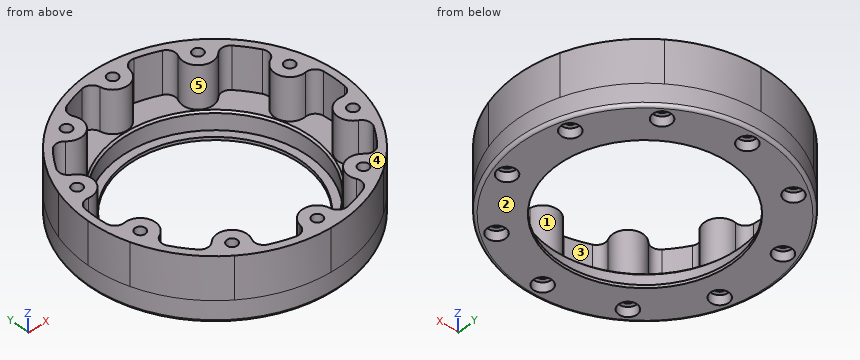
from build123d import *
from build123d.topology import SkipClean

# Parameters (mm, degrees)
ESQUISSE1_R             = 42
ESQUISSE1_R_2           = 31.2
BOSS_EXTRU_1_DEPTH      = 6
BOSS_EXTRU_2_START      = 1
ESQUISSE2_R             = 42
ESQUISSE2_R_2           = 28.6
BOSS_EXTRU_2_DEPTH      = 1
ESQUISSE3_R             = 5
BOSS_EXTRU_3_DEPTH      = 14
ESQUISSE4_R             = 42
ESQUISSE4_R_2           = 39.6
BOSS_EXTRU_4_DEPTH      = 14
CONG_1_R                = 3
ESQUISSE5_R             = 1.7
ENL_V_MAT_EXTRU_1_DEPTH = 64.000000167
ESQUISSE6_R             = 3
ENL_V_MAT_EXTRU_2_DEPTH = 3.2
CHANFREIN1_SIZE         = 0.6
CONG_2_R                = 1


with BuildPart() as part:
    # Esquisse1 → Boss.-Extru.1 (new body)
    with BuildSketch(Plane.XY):
        Circle(ESQUISSE1_R)
        Circle(ESQUISSE1_R_2, mode=Mode.SUBTRACT)
    extrude(amount=BOSS_EXTRU_1_DEPTH)

    # Esquisse2 → Boss.-Extru.2 (add)
    with BuildSketch(Plane(origin=(0, 0, 0), x_dir=(-1, 0, 0), z_dir=(0, 0, -1)).offset(BOSS_EXTRU_2_START)):
        Circle(ESQUISSE2_R)
        Circle(ESQUISSE2_R_2, mode=Mode.SUBTRACT)
    extrude(amount=-BOSS_EXTRU_2_DEPTH)

    # Esquisse3 → Boss.-Extru.3 (add)
    with BuildSketch(Plane.XY.offset(6)):
        with Locations(Location((0, 37, 0), (0, 0, 89.999613921))):
            Circle(ESQUISSE3_R)
        with Locations(Location((21.748054335, 29.933628792, 0), (0, 0, 53.999609041))):
            Circle(ESQUISSE3_R)
        with Locations(Location((35.189091103, 11.433628792, 0), (0, 0, 17.999603008))):
            Circle(ESQUISSE3_R)
        with Locations(Location((35.189091103, -11.433628792, 0), (0, 0, 341.999598271))):
            Circle(ESQUISSE3_R)
        with Locations(Location((21.748054335, -29.933628792, 0), (0, 0, 305.999596518))):
            Circle(ESQUISSE3_R)
        with Locations(Location((0, -37, 0), (0, 0, 269.999598257))):
            Circle(ESQUISSE3_R)
        with Locations(Location((-21.748054335, -29.933628792, 0), (0, 0, 233.999602875))):
            Circle(ESQUISSE3_R)
        with Locations(Location((-35.189091103, -11.433628792, 0), (0, 0, 197.999608525))):
            Circle(ESQUISSE3_R)
        with Locations(Location((-35.189091103, 11.433628792, 0), (0, 0, 161.99961318))):
            Circle(ESQUISSE3_R)
        with Locations(Location((-21.748054335, 29.933628792, 0), (0, 0, 125.999614883))):
            Circle(ESQUISSE3_R)
    extrude(amount=BOSS_EXTRU_3_DEPTH)

    # Esquisse4 → Boss.-Extru.4 (add)
    with SkipClean():  # the faces are left unmerged after this step: merging them gives an invalid solid
        with BuildSketch(Plane.XY.offset(6)):
            with Locations(Location((0, 0, 0), (0, 0, 180))):
                Circle(ESQUISSE4_R)
            Circle(ESQUISSE4_R_2, mode=Mode.SUBTRACT)
        extrude(amount=BOSS_EXTRU_4_DEPTH)

    # Congé1
    cong_1_edges = [part.edges().sort_by_distance(p)[0] for p in [
        (-4.411459412, 39.353513514, 13),
        (4.411459412, 39.353513514, 13),
        (19.562469235, 34.430652004, 13),
        (26.700360503, 29.244670437, 13),
        (36.064199538, 16.356451684, 13),
        (38.790631394, 7.965357244, 13),
        (38.790631394, -7.965357244, 13),
        (36.064199538, -16.356451684, 13),
        (26.700360503, -29.244670437, 13),
        (19.562469235, -34.430652004, 13),
        (4.411459412, -39.353513514, 13),
        (-4.411459412, -39.353513514, 13),
        (-19.562469235, -34.430652004, 13),
        (-26.700360503, -29.244670437, 13),
        (-36.064199538, -16.356451684, 13),
        (-38.790631394, -7.965357244, 13),
        (-38.790631394, 7.965357244, 13),
        (-36.064199538, 16.356451684, 13),
        (-26.700360503, 29.244670437, 13),
        (-19.562469235, 34.430652004, 13),
    ]]
    fillet(cong_1_edges, radius=CONG_1_R)

    # Esquisse5 → Enlèv. mat.-Extru.1 (cut, through all)
    with BuildSketch(Plane(origin=(0, 0, -1), x_dir=(-1, 0, 0), z_dir=(0, 0, -1))):
        with Locations((0, 37)):
            Circle(ESQUISSE5_R)
        with Locations((21.748054335, 29.933628792)):
            Circle(ESQUISSE5_R)
        with Locations((35.189091103, 11.433628792)):
            Circle(ESQUISSE5_R)
        with Locations((35.189091103, -11.433628792)):
            Circle(ESQUISSE5_R)
        with Locations((21.748054335, -29.933628792)):
            Circle(ESQUISSE5_R)
        with Locations((0, -37)):
            Circle(ESQUISSE5_R)
        with Locations((-21.748054335, -29.933628792)):
            Circle(ESQUISSE5_R)
        with Locations((-35.189091103, -11.433628792)):
            Circle(ESQUISSE5_R)
        with Locations((-35.189091103, 11.433628792)):
            Circle(ESQUISSE5_R)
        with Locations((-21.748054335, 29.933628792)):
            Circle(ESQUISSE5_R)
    extrude(amount=-ENL_V_MAT_EXTRU_1_DEPTH, mode=Mode.SUBTRACT)

    # Esquisse6 → Enlèv. mat.-Extru.2 (cut)
    with BuildSketch(Plane(origin=(0, 0, -1), x_dir=(-1, 0, 0), z_dir=(0, 0, -1))):
        with Locations((0, 37)):
            Circle(ESQUISSE6_R)
        with Locations((21.748054335, 29.933628792)):
            Circle(ESQUISSE6_R)
        with Locations((35.189091103, 11.433628792)):
            Circle(ESQUISSE6_R)
        with Locations((35.189091103, -11.433628792)):
            Circle(ESQUISSE6_R)
        with Locations((21.748054335, -29.933628792)):
            Circle(ESQUISSE6_R)
        with Locations((0, -37)):
            Circle(ESQUISSE6_R)
        with Locations((-21.748054335, -29.933628792)):
            Circle(ESQUISSE6_R)
        with Locations((-35.189091103, -11.433628792)):
            Circle(ESQUISSE6_R)
        with Locations((-35.189091103, 11.433628792)):
            Circle(ESQUISSE6_R)
        with Locations((-21.748054335, 29.933628792)):
            Circle(ESQUISSE6_R)
    extrude(amount=-ENL_V_MAT_EXTRU_2_DEPTH, mode=Mode.SUBTRACT)

    # Chanfrein1
    chanfrein1_edges = [part.edges().sort_by_distance(p)[0] for p in [
        (-31.2, 0, 6),
    ]]
    chamfer(chanfrein1_edges, length=CHANFREIN1_SIZE)

    # Congé2
    cong_2_edges = [part.edges().sort_by_distance(p)[0] for p in [
        (42, 0, -1),
    ]]
    fillet(cong_2_edges, radius=CONG_2_R - 0.0001)  # a hair under: the kernel refuses the full size


solid = part.part
Verification items for the finished model (mm, model axes). Face numbers are marked on the shaded views. A direction names the side the tool comes from. Coordinates: 2 decimals unless noted, no trailing zeros. Write each question's results on one line, items separated by ' | '.
1) Section check A-A on z = 15.75. Give the number of separate pieces and of enclosed holes in the cut face, plus the area to 3 significant figures.
Solved:
separate pieces: 1 | enclosed holes: 11 | area: 1,220 mm²
2) Scan lines: line 1 along Y through (x, z) = (0, 9); line 2 along X through (y, z) = (-32.5, 6.25); line 3 along X through (y, z) = (0.5, 18.5). Record each from-to range of solid material in increasing order. Write a range as [from, to].
Solved:
line 1: y = [-42, -38.7], [-35.3, -32], [32, 35.3], [38.7, 42] | line 2: x = [-26.6, -17.42], [-2.18, 2.18], [17.42, 26.6] | line 3: x = [-42, -39.6], [39.6, 42]
3) Release check for a two-part mould opening along Y. For the marked faces 1, 2 and 3 record: pulls with the +Y half, pulls with the -Y half, needs draft (parallel to the pull), parting line crosses it, or undercut.
Solved:
face 1: undercut | face 2: needs draft | face 3: undercut
4) Access from +Z, -Z, +X, -X, +Y, -Y to the whole of each face (thin tool, end or side, straight path). Record for the marked faces 4 and 5.
Solved:
face 4: +Z, +X, -X, +Y, -Y | face 5: +Z
5) Gauge pin test, flat ends, axial feed: pin 1 Ø3 at (x, y) = (22.5, -30.5) entering from -Z; pin 2 Ø5 at (x, z) = (32, 12.5) entering from -Y; pin 3 Ø12 at (x, z) = (-19.5, 9) entering from -Y; pin 4 Ø2 at (x, y) = (21.75, 29.93) entering from +Z. Record the tip position at first contact, or that the pin passes through.
Solved:
pin 1: stops at z = 2.2 | pin 2: stops at y = -29.9 | pin 3: stops at y = -39.77 | pin 4: passes through
